The model under review builds one solid part; all positions refer to its coordinate system, in mm. A direction names the side the tool comes from. Coordinates: 2 decimals unless noted, no trailing zeros. Loops run counter-clockwise (first coordinate to the right, second up) from the corner with the lowest first, then second, coordinate; pieces in that order, holes last. Notation, with made-up numbers: M 84,-30 L 89,-30 A20 ccw 89,-5 Z; hole C 25.25,-11.5 d7. An arc over 180 degrees is marked long. Use one line per item in the form item = value.
```python
from build123d import *

# Parameters (mm, degrees)
SKIZZE1_R                         = 15
AUFSATZ_LINEAR_AUSTRAGEN1_DEPTH   = 30
SKIZZE1_W                         = 30
SKIZZE1_H                         = 30
AUFSATZ_LINEAR_AUSTRAGEN1_2_DEPTH = 30
AUFSATZ_LINEAR_AUSTRAGEN1_3_DEPTH = 30
SKIZZE1_H_2                       = 15
AUFSATZ_LINEAR_AUSTRAGEN1_4_DEPTH = 30
AUFSATZ_LINEAR_AUSTRAGEN1_5_DEPTH = 30
LINEAR_AUSTRAGEN_D_NN1_DEPTH      = 0.4


with BuildPart() as part:
    # Skizze1 → Aufsatz-Linear austragen1 (new body)
    with BuildSketch(Plane(origin=(0, 0, 0), x_dir=(1, 0, 0), z_dir=(0, 1, 0))):
        with Locations((-10, 0)):
            Circle(SKIZZE1_R)
    extrude(amount=AUFSATZ_LINEAR_AUSTRAGEN1_DEPTH)



with BuildPart() as body_2:
    # Skizze1 → Aufsatz-Linear austragen1 2 (new body)
    with BuildSketch(Plane(origin=(0, 0, 0), x_dir=(1, 0, 0), z_dir=(0, 1, 0))):
        with Locations((30, 20)):
            Rectangle(SKIZZE1_W, SKIZZE1_H)
    extrude(amount=AUFSATZ_LINEAR_AUSTRAGEN1_2_DEPTH)


with BuildPart() as body_3:
    # Skizze1 → Aufsatz-Linear austragen1 3 (new body)
    with BuildSketch(Plane(origin=(0, 0, 0), x_dir=(1, 0, 0), z_dir=(0, 1, 0))):
        Polygon((38.660254038, -5), (21.339745962, -5), (12.679491924, -20), (21.339745962, -35), (38.660254038, -35), (47.320508076, -20), align=None)
    extrude(amount=AUFSATZ_LINEAR_AUSTRAGEN1_3_DEPTH)


with BuildPart() as body_4:
    # Skizze1 → Aufsatz-Linear austragen1 4 (new body)
    with BuildSketch(Plane(origin=(0, 0, 0), x_dir=(1, 0, 0), z_dir=(0, 1, 0))):
        with Locations((70, 20)):
            Rectangle(SKIZZE1_W, SKIZZE1_H_2)
    extrude(amount=AUFSATZ_LINEAR_AUSTRAGEN1_4_DEPTH)


with BuildPart() as body_5:
    # Skizze1 → Aufsatz-Linear austragen1 5 (new body)
    with BuildSketch(Plane(origin=(0, 0, 0), x_dir=(1, 0, 0), z_dir=(0, 1, 0))):
        Polygon((76.213203436, -5), (63.786796564, -5), (55, -13.786796564), (55, -26.213203436), (63.786796564, -35), (76.213203436, -35), (85, -26.213203436), (85, -13.786796564), align=None)
    extrude(amount=AUFSATZ_LINEAR_AUSTRAGEN1_5_DEPTH)


with BuildPart() as part_1:
    add(part.part)

    add(body_2.part)  # Linear-Austragen-D_nn1 merges body 2

    add(body_3.part)  # Linear-Austragen-D_nn1 merges body 3

    add(body_4.part)  # Linear-Austragen-D_nn1 merges body 4

    add(body_5.part)  # Linear-Austragen-D_nn1 merges body 5
    # Skizze2 → Linear-Austragen-D_nn1 (add)
    with BuildSketch(Plane.XZ):
        Polygon((29.905572809, 20.4), (-10.894427191, 0), (29.905572809, -20.4), (70.4, -20.4), (70.4, 20.4), align=None)
        Polygon((30.094427191, 19.6), (-9.105572809, 0), (30.094427191, -19.6), (69.6, -19.6), (69.6, 19.6), align=None, mode=Mode.SUBTRACT)
    extrude(amount=-LINEAR_AUSTRAGEN_D_NN1_DEPTH)


solid = part_1.part
```
1. Insertion check: P1, Ø5, axis at x = 65.5, y = 23.5, coming from the -Z side; P2, Ø2, axis at x = 14.5, y = 23.5, coming from the +Z side; P3, Ø15, axis at y = 14.5, z = -14, coming from the -X side; P4, Ø7.5, axis at x = 11.5, z = -8.5, coming from the +Y side. Each pin has a flat end and moves straight along its axis. Give the tip position at first contact, or say it passes through.
Response values:
P1 = -27.5
P2 = 24.89
P3 = -23.52
P4 = 30
2. Add section A-A (z = -22.5). State the section outline as (x, y) points.
Response values:
outline = M 15,0 L 45,0 L 45,30 L 15,30 Z; M 55,0 L 85,0 L 85,30 L 55,30 Z
3. Wall thickness on line 1 along X through (y, z) = (8, -15.5); line 2 along Z through (x, y) = (70.5, 4.5); line 3 along X through (y, z) = (7.5, 13.5): over which ranges is each line inside the solid? List them lowest first. Write a range as from..to.
Response values:
line_1 = 15..45, 55..85
line_2 = -27.5..-12.5, 5..35
line_3 = -16.54..-3.46, 16.43..43.57, 55.29..84.71
4. Add section C-C (y = 6.75). State the section outline as (x, z) points.
Response values:
outline = C -10,0 d30; M 12.68,20 L 21.34,5 L 38.66,5 L 47.32,20 L 38.66,35 L 21.34,35 Z; M 15,-35 L 45,-35 L 45,-5 L 15,-5 Z; M 55,-27.5 L 85,-27.5 L 85,-12.5 L 55,-12.5 Z; M 55,13.79 L 63.79,5 L 76.21,5 L 85,13.79 L 85,26.21 L 76.21,35 L 63.79,35 L 55,26.21 Z
5. Machinability: for faces 1 (the face through (59.455, 14.79, 9.332)), 2 (the face through (29, 0, 7)), 3 (the face through (9.03, 0.2, -9.96)), which of the approach directions +Z, -Z, +X, -X, +Y, -Y give a long, thin tool a straight path to every point of the face, cutting with its end or side? Answer none if there is none.
Response values:
face_1 = +Y, -Y
face_2 = +Z, -Z, +X, -X, -Y
face_3 = -Z, +Y, -Y
6. The part is to be moulded in two halves that separate along X. For faces 4 (the face through (70, 30, 20)), 5 (the face through (45, 15, -20)), 6 (the face through (85, 15, 20)), say which applies: pulls with the +X half, pulls with the -X half, needs draft (parallel to the pull), parting line crosses it, or undercut.
Response values:
face_4 = needs draft
face_5 = undercut
face_6 = pulls with the +X half
7. Add section B-B (x = 29.5). State the section outline as (y, z) points, then the cut area to 3 significant figures.
Response values:
outline = M 0,-35 L 30,-35 L 30,-5 L 0,-5 Z; M 0,5 L 30,5 L 30,35 L 0,35 Z
area = 1,800 mm^2
8. Add section D-D (z = 10.5). State the section outline as (x, y) points, then the cut area to 3 significant figures.
Response values:
outline = M -20.71,0 L 0.71,0 L 0.71,30 L -20.71,30 Z; M 10.11,0 L 11.89,0 L 11.89,0.4 L 10.11,0.4 Z; M 18.16,0 L 41.84,0 L 41.84,30 L 18.16,30 Z; M 58.29,0 L 81.71,0 L 81.71,30 L 58.29,30 Z
area = 2,060 mm^2
